from build123d import *

# Parameters (mm, degrees)
SKETCH_1_R          = 6
EXTRUDE_1_DEPTH     = 3
SKETCH_2_R          = 6
EXTRUDE_2_DEPTH     = 13
HOLE_WIZARD_M6_1_D  = 5
SKETCH_6_R          = 3
CUT_EXTRUDE_1_DEPTH = 10


with BuildPart() as part:
    # 草图1 → 凸台-拉伸1 (new body)
    with BuildSketch(Plane(origin=(0, 0, 0), x_dir=(1, 0, 0), z_dir=(0, 1, 0))):
        with Locations((-13.5, 0)):
            Circle(SKETCH_1_R)
        with BuildLine():
            Line((13.5, 6), (-13.5, 6))
            ThreePointArc((-13.5, 6), (-9.257359313, 4.242640687), (-7.5, 0))
            ThreePointArc((-7.5, 0), (-9.257359313, -4.242640687), (-13.5, -6))
            Line((-13.5, -6), (13.5, -6))
            ThreePointArc((13.5, -6), (7.5, 0), (13.5, 6))
        make_face()
        with Locations((13.5, 0)):
            Circle(SKETCH_1_R)
        with BuildLine():
            Line((-13.5, -6), (-13.5, 6))
            ThreePointArc((-13.5, 6), (-19.5, 0), (-13.5, -6))
        make_face()
        with BuildLine():
            ThreePointArc((19.5, 0), (17.742640687, 4.242640687), (13.5, 6))
            Line((13.5, 6), (13.5, -6))
            ThreePointArc((13.5, -6), (17.742640687, -4.242640687), (19.5, 0))
        make_face()
    extrude(amount=EXTRUDE_1_DEPTH)

    # 草图2 → 凸台-拉伸2 (add)
    with BuildSketch(Plane(origin=(0, 3, 0), x_dir=(1, 0, 0), z_dir=(0, 1, 0))):
        Circle(SKETCH_2_R)
    extrude(amount=EXTRUDE_2_DEPTH)

    # M6 螺纹孔1 (through all)
    with Locations(Plane(origin=(0, 16, 0), x_dir=(1, 0, 0), z_dir=(0, 1, 0))):
        with Locations((0, 0)):
            Hole(HOLE_WIZARD_M6_1_D / 2)

    # 草图6 → 切除-拉伸1 (cut)
    with BuildSketch(Plane(origin=(0, 3, 0), x_dir=(1, 0, 0), z_dir=(0, 1, 0))):
        with Locations((-13.5, 0)):
            Circle(SKETCH_6_R)
        with Locations((13.5, 0)):
            Circle(SKETCH_6_R)
    extrude(amount=-CUT_EXTRUDE_1_DEPTH, mode=Mode.SUBTRACT)


solid = part.part
CAD build for the part. Positions are in the model's coordinates, mm. Round coordinates to 2 decimals unless told otherwise and drop trailing zeros. Write each loop counter-clockwise with the first axis right and the second up, starting at its lowest first coordinate (ties: lowest second). Pieces come first, ordered by that corner, then holes.
(1) Slice it at B-B, the plane y = 1.5. Write the cut outline in (x, z).
(2) Drop flat-ended pins along their axis: P1, Ø4.5, axis at x = 0, z = 0, coming from the +Y side; P2, Ø3.5, axis at x = 8.5, z = -1.5, coming from the +Y side; P3, Ø2, axis at y = 3, z = -1, coming from the -X side; P4, Ø2, axis at y = 6, z = 2.5, coming from the +X side. Give the stop position or say it passes through.
(3) Slice it at C-C, the plane x = 11. Write the cut outline in (y, z), and give its area (3 significant figures).
(4) Slice it at D-D, the plane y = 7.25. Write the cut outline in (x, z).
(5) Slice it at A-A, the plane z = 0. Write the cut outline in (x, y).
(6) Probe line 1 along Z through (x, y) = (-13.5, 2.1); line 2 along Z through (x, y) = (0, 4); line 3 along Y through (x, z) = (8, 4.5). List the from-to ranges inside material, lowest first.
(7) Mould opens along X. For faces 1 (the face through (19.5, 1.5, 0.1)), 2 (the face through (0.54, 7.89, 2.44)), 3 (the face through (-6, 9, 0)) say: pulls with the +X half, pulls with the -X half, needs draft (parallel to the pull), parting line crosses it, or undercut.
From the geometry:
1. outline: (-13.5, -6) - (13.5, -6) arc R6 ccw to (13.5, 6) - (-13.5, 6) arc R6 ccw to start; hole circle Ø6 at (-13.5, 0); hole circle Ø5 at (0, 0); hole circle Ø6 at (13.5, 0)
2. P1: passes through
2. P2: stops at y = 3
2. P3: stops at x = -19.5
2. P4: stops at x = 5.81
3. outline: (0, -6) - (3, -6) - (3, -1.66) - (0, -1.66) - close; (0, 1.66) - (3, 1.66) - (3, 6) - (0, 6) - close
3. area: 26.1 mm2
4. outline: circle Ø12 at (0, 0); hole circle Ø5 at (0, 0)
5. outline: (-19.5, 0) - (-16.5, 0) - (-16.5, 3) - (-19.5, 3) - close; (-10.5, 0) - (-2.5, 0) - (-2.5, 16) - (-6, 16) - (-6, 3) - (-10.5, 3) - close; (2.5, 0) - (10.5, 0) - (10.5, 3) - (6, 3) - (6, 16) - (2.5, 16) - close; (16.5, 0) - (19.5, 0) - (19.5, 3) - (16.5, 3) - close
6. line 1: z = -6 to -3, 3 to 6
6. line 2: z = -6 to -2.5, 2.5 to 6
6. line 3: y = 0 to 3
7. face 1: pulls with the +X half
7. face 2: undercut
7. face 3: parting line crosses it
